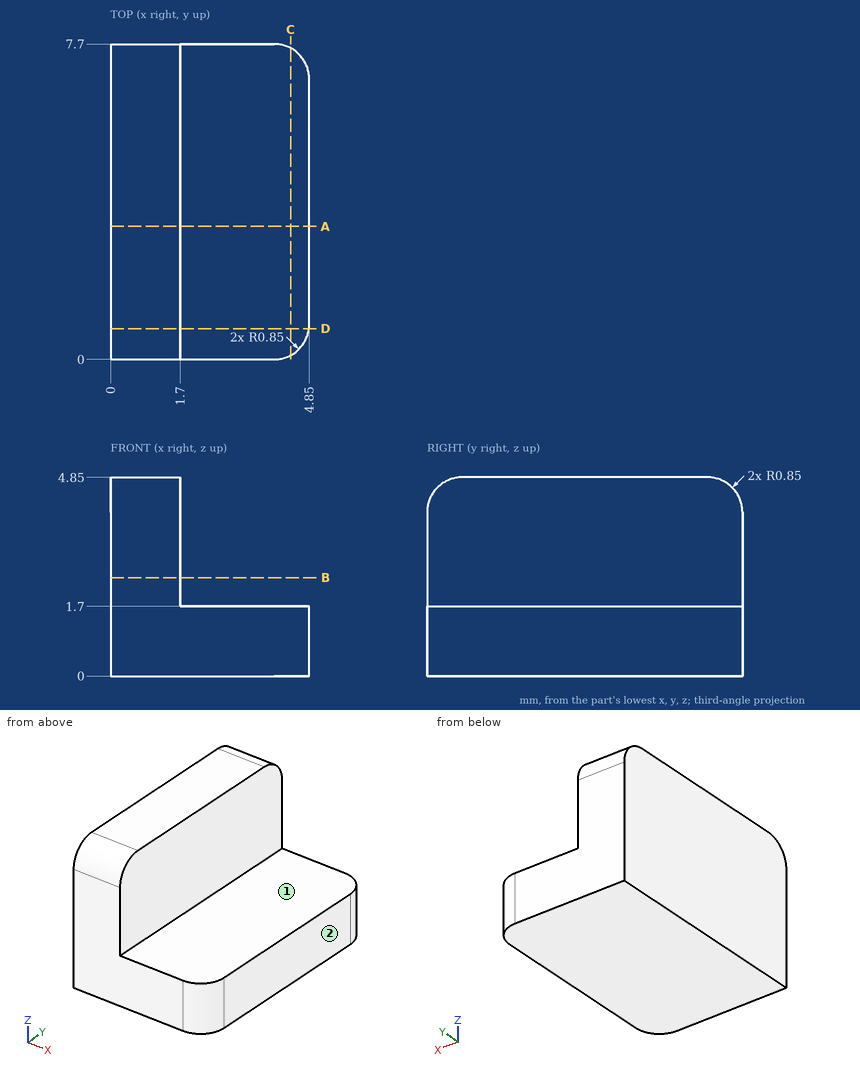
Design review of the part shown in the three views and the two pictorial views. Dimensions are in mm from the part's minimum x, y and z. A direction names the side the tool comes from. Give positions to 0.01 mm unless a question says otherwise; leave off trailing zeros. Write each loop counter-clockwise with the first axis right and the second up, starting at its lowest first coordinate (ties: lowest second). Pieces come first, ordered by that corner, then holes. Notation, with made-up numbers: M -23.75,48.25 L 33.25,48.25 A37 cw 33.25,84.25 Z; hole C 44,84 d2. An arc over 180 degrees is marked long. Answer in a Markdown table with one row per item.
Item 1: For line 1 along X through (y, z) = (7, 4); line 2 along X through (y, z) = (0.75, 0.55), list the stretches that pass through material, from the lowest coordinate up.
Check sheet entries:
| item | result |
|---|---|
| line 1 | 0 to 1.7 |
| line 2 | 0 to 4.84 |
Item 2: Add section D-D on y = 0.75. Give the boundary of the cut face in (x, z).
Check sheet entries:
| item | result |
|---|---|
| outline | M 0,0 L 4.84,0 L 4.84,1.7 L 1.7,1.7 L 1.7,4.84 L 0,4.84 Z |
Item 3: Add section B-B on z = 2.4. Give the boundary of the cut face in (x, y), plus the area to 3 significant figures.
Check sheet entries:
| item | result |
|---|---|
| outline | M 0,0 L 1.7,0 L 1.7,7.7 L 0,7.7 Z |
| area | 13.1 mm2 |
Item 4: Add section A-A on y = 3.25. Give the boundary of the cut face in (x, z).
Check sheet entries:
| item | result |
|---|---|
| outline | M 0,0 L 4.85,0 L 4.85,1.7 L 1.7,1.7 L 1.7,4.85 L 0,4.85 Z |
Item 5: Tool access review of the marked faces 1 and 2: name each direction out of +Z, -Z, +X, -X, +Y, -Y from which nothing blocks a thin tool from reaching the whole face with its end or side.
Check sheet entries:
| item | result |
|---|---|
| face 1 | +Z, +X, +Y, -Y |
| face 2 | +Z, -Z, +X, +Y, -Y |
Item 6: Add section C-C on x = 4.4. Give the boundary of the cut face in (y, z).
Check sheet entries:
| item | result |
|---|---|
| outline | M 0.1,0 L 7.6,0 L 7.6,1.7 L 0.1,1.7 Z |
Item 7: For P1, Ø2.5, axis at y = 3, z = 4, coming from the +X side, flat-tipped, find the tip position at first contact; note if it passes through.
Check sheet entries:
| item | result |
|---|---|
| P1 | x = 1.7 |
